For this review, take the finished solid that the model builds, in its own axes (mm). A direction names the side the tool comes from. Round coordinates to 2 decimals unless told otherwise and drop trailing zeros. Order: outer loops, then holes, each group sorted by start corner. A loop starts at its lowest first (then second) coordinate and runs counter-clockwise, first axis right, second up. Notation, with made-up numbers: (85.25, -13) - (100.25, -13) arc R22 cw to (100.25, 10) - close; hole circle Ø2 at (8, 37.25). An arc over 180 degrees is marked (long way). One line per item, written item: value.
```python
from build123d import *

# Parameters (mm, degrees)
SKETCH_1_W               = 50
SKETCH_1_H               = 40
EXTRUDE_2_DEPTH          = 47
SKETCH_3_W               = 70
SKETCH_3_H               = 10
EXTRUDE_3_DEPTH          = 10
CUT_EXTRUDE_1_DEPTH      = 62.919302322
CUT_EXTRUDE_1_DEPTH_BACK = 62.919302322
SKETCH_4_R               = 11.5
SKETCH_5_W               = 39
SKETCH_5_H               = 36
CUT_EXTRUDE_2_DEPTH      = 43.5
M3X0_5_1_D               = 2.5
SKETCH_8_W               = 39
SKETCH_8_H               = 70
CUT_EXTRUDE_3_DEPTH      = 35


with BuildPart() as part:
    # ｽｹｯﾁ1 → ﾎﾞｽ - 押し出し2 (new body)
    with BuildSketch(Plane.XY):
        Rectangle(SKETCH_1_W, SKETCH_1_H)
    extrude(amount=EXTRUDE_2_DEPTH)

    # ｽｹｯﾁ3 → ﾎﾞｽ - 押し出し3 (add)
    with BuildSketch(Plane.XY):
        with Locations((0, -15)):
            Rectangle(SKETCH_3_W, SKETCH_3_H)
    extrude_3 = extrude(amount=EXTRUDE_3_DEPTH)

    # ｽｹｯﾁ4 → ｶｯﾄ - 押し出し1 (cut, two sides: drawn at the far end of the back side and taken through both)
    with BuildSketch(Plane.XY.offset(-CUT_EXTRUDE_1_DEPTH_BACK)):
        Circle(SKETCH_4_R)
    extrude(amount=CUT_EXTRUDE_1_DEPTH + CUT_EXTRUDE_1_DEPTH_BACK, mode=Mode.SUBTRACT)

    # ｽｹｯﾁ5 → ｶｯﾄ - 押し出し2 (cut)
    with BuildSketch(Plane.XY):
        Rectangle(SKETCH_5_W, SKETCH_5_H)
    cut_extrude_2 = extrude(amount=CUT_EXTRUDE_2_DEPTH, mode=Mode.SUBTRACT)

    # M3x0.5 ねじ穴1 (through all)
    with Locations(Plane.XY.offset(10)):
        with Locations((30, -15), (-30, -15)):
            m3x0_5_1 = Hole(M3X0_5_1_D / 2)

    # ｽｹｯﾁ8 → ｶｯﾄ - 押し出し3 (cut)
    with BuildSketch(Plane(origin=(0, 0, 0), x_dir=(-1, 0, 0), z_dir=(0, 0, -1))):
        Rectangle(SKETCH_8_W, SKETCH_8_H)
    cut_extrude_3 = extrude(amount=-CUT_EXTRUDE_3_DEPTH, mode=Mode.SUBTRACT)

    # ﾐﾗｰ4: ﾎﾞｽ - 押し出し3, ｶｯﾄ - 押し出し2, M3x0.5 ねじ穴1, ｶｯﾄ - 押し出し3 across plane
    add(extrude_3.mirror(Plane.ZX))
    add(cut_extrude_2.mirror(Plane.ZX), mode=Mode.SUBTRACT)
    add(m3x0_5_1.mirror(Plane.ZX), mode=Mode.SUBTRACT)
    add(cut_extrude_3.mirror(Plane.ZX), mode=Mode.SUBTRACT)


solid = part.part
```
Item 1: Take a section at C-C (z = 6.5). Write out the cut boundary in (x, y), plus the area to 3 significant figures.
Returned:
outline: (-35, -20) - (-19.5, -20) - (-19.5, 20) - (-35, 20) - (-35, 10) - (-25, 10) - (-25, -10) - (-35, -10) - close; (19.5, -20) - (35, -20) - (35, -10) - (25, -10) - (25, 10) - (35, 10) - (35, 20) - (19.5, 20) - close; hole circle Ø2.5 at (-30, -15); hole circle Ø2.5 at (-30, 15); hole circle Ø2.5 at (30, -15); hole circle Ø2.5 at (30, 15)
area: 820 mm^2
Item 2: Machinability: for faces 1 (the flat face through (-29, -16, 10)), 2 (the flat face through (31, -16, 10)), 3 (the flat face through (-30, 10, 5)), 4 (the flat face through (0, -19, 35)), which of the approach directions +Z, -Z, +X, -X, +Y, -Y give a long, thin tool a straight path to every point of the face, cutting with its end or side? Answer none if there is none.
Returned:
face 1: +Z, -X, +Y, -Y
face 2: +Z, +X, +Y, -Y
face 3: +Z, -Z, -X
face 4: -Z, +Y, -Y
Item 3: Take a section at A-A (y = 0). Write out the cut boundary in (x, z), plus the area to 3 significant figures.
Returned:
outline: (-25, 0) - (-19.5, 0) - (-19.5, 43.5) - (-11.5, 43.5) - (-11.5, 47) - (-25, 47) - close; (11.5, 43.5) - (19.5, 43.5) - (19.5, 0) - (25, 0) - (25, 47) - (11.5, 47) - close
area: 573 mm^2
Item 4: Take a section at D-D (z = 40). Write out the cut boundary in (x, y).
Returned:
outline: (-25, -20) - (25, -20) - (25, 20) - (-25, 20) - close; hole (-19.5, -18) - (19.5, -18) - (19.5, 18) - (-19.5, 18) - close
Item 5: For P1, Ø2, axis at x = -30, y = -15, coming from the +Z side; P2, Ø12, axis at y = 7, z = 18, coming from the +X side; P3, Ø1.6, axis at x = 4, y = 19, coming from the -Z side; P4, Ø12, axis at y = -7, z = 18, coming from the -X side, all flat-tipped, find the tip position at first contact; note any pin that passes through.
Returned:
P1: through
P2: x = 25
P3: z = 35
P4: x = -25
Item 6: The part is to be moulded in two halves that separate along X. For faces 5 (the cylindrical face through (29.328, 13.946, 4.93)), 6 (the flat face through (0, 20, 39)), say which applies: +X half, -X half, draft (parallel to the pull), parting line (faces both ways), or undercut.
Returned:
face 5: undercut
face 6: draft
Item 7: Take a section at B-B (x = 30). Write out the cut boundary in (y, z), plus the area to 3 significant figures.
Returned:
outline: (-20, 0) - (-16.25, 0) - (-16.25, 10) - (-20, 10) - close; (-13.75, 0) - (-10, 0) - (-10, 10) - (-13.75, 10) - close; (10, 0) - (13.75, 0) - (13.75, 10) - (10, 10) - close; (16.25, 0) - (20, 0) - (20, 10) - (16.25, 10) - close
area: 150 mm^2
Item 8: Wall thickness on line 1 (Y direction, x = 30, z = 8); line 2 (X direction, y = 11, z = 36); line 3 (Z direction, x = 19, y = -12): over which ranges is each line inside the solid? List them lowest first.
Returned:
line 1: -20 to -16.25, -13.75 to -10, 10 to 13.75, 16.25 to 20
line 2: -25 to -19.5, 19.5 to 25
line 3: 43.5 to 47
